from build123d import *

# Parameters (mm, degrees)
F0_W     = 113.03
F0_H     = 34.544
F1_DEPTH = 14.605
F3_DEPTH = 34.545


with BuildPart() as f1:
    # F0 (on Top) → F1 (new body, symmetric)
    with BuildSketch(Plane.XY):
        Rectangle(F0_W, F0_H)
    extrude(amount=F1_DEPTH, both=True)

    # F2 (on face) → F3 (cut, through all)
    with BuildSketch(Plane.XZ.offset(17.272)):
        with BuildLine():
            ThreePointArc((50.165, 14.605), (54.858827, 7.962859), (56.515, 0))
            Line((56.515, 0), (56.515, 14.605))
            Line((56.515, 14.605), (50.165, 14.605))
        make_face()
        with BuildLine():
            ThreePointArc((56.515, 0), (54.858827, -7.962859), (50.165, -14.605))
            Line((50.165, -14.605), (56.515, -14.605))
            Line((56.515, -14.605), (56.515, 0))
        make_face()
    extrude(amount=-F3_DEPTH, mode=Mode.SUBTRACT)


solid = f1.part
Source: CAD feature listing. Evaluate the final solid. Frame: model axes, mm. Give positions to 0.01 mm unless a question says otherwise; leave off trailing zeros. Write each loop counter-clockwise with the first axis right and the second up, starting at its lowest first coordinate (ties: lowest second). Pieces come first, ordered by that corner, then holes. Notation, with made-up numbers: M 24,26 L 61,26 A10 cw 61,34 Z; hole C 37,54 d1. An arc over 180 degrees is marked long. Answer as a JSON object with one key per item and string values.
Q1. Cut plane A-A, the plane y = -2.5. Return the cut outline in (x, z) (1 decimal).
Geometry check:
{"outline": "M -56.5,-14.6 L 50.2,-14.6 A20 ccw 50.2,14.6 L -56.5,14.6 Z"}
Q2. Ray query, line 1 along X through (y, z) = (11, 11.25) (3 decimals); line 2 along X through (y, z) = (-11, -10.75) (3 decimals). Return the intervals inside material, ascending.
Geometry check:
{"line 1": "x = -56.515 to 53.045", "line 2": "x = -56.515 to 53.375"}
Q3. Cut plane C-C, the plane z = -9.25. Return the cut outline in (x, y) (3 decimals).
Geometry check:
{"outline": "M -56.515,-17.272 L 54.244,-17.272 L 54.244,17.272 L -56.515,17.272 Z"}
Q4. Cut plane B-B, the plane z = 12. Return the cut outline in (x, y) (3 decimals), then the cut area to 3 significant figures.
Geometry check:
{"outline": "M -56.515,-17.272 L 52.508,-17.272 L 52.508,17.272 L -56.515,17.272 Z", "area": "3,770 mm^2"}
